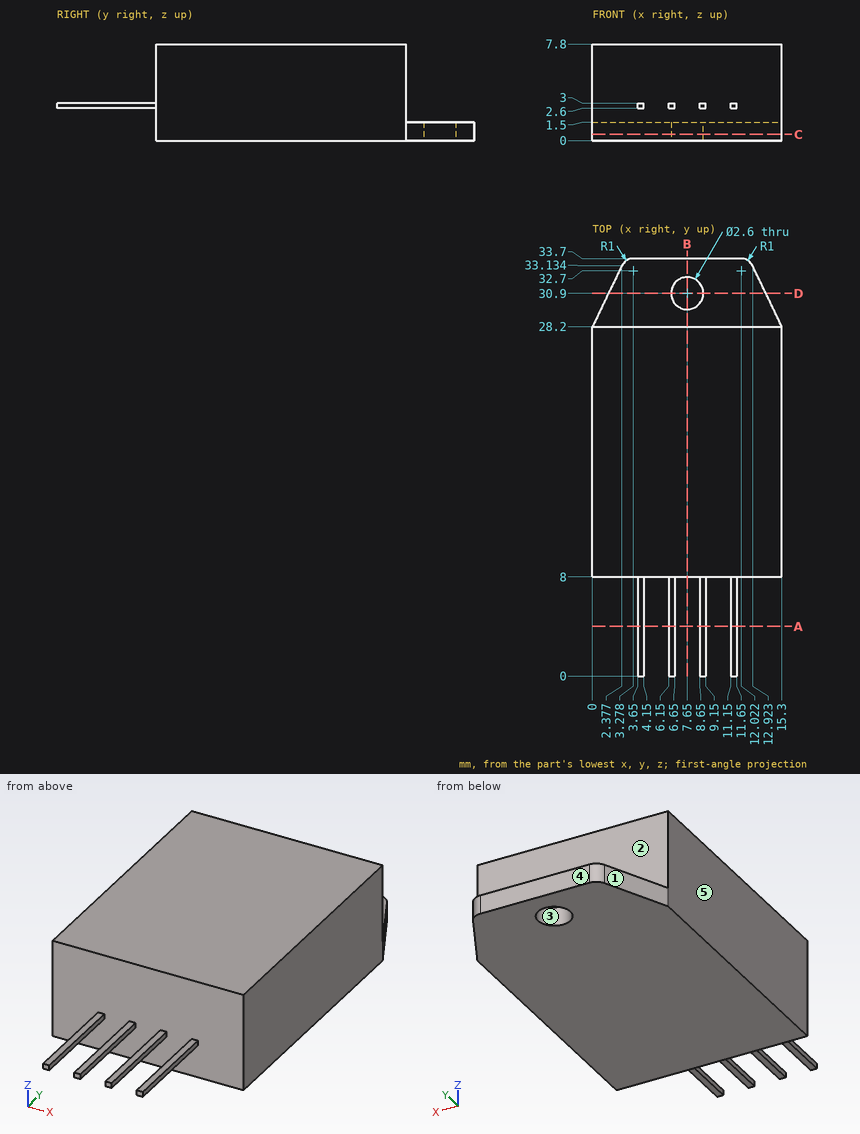
Can you work these out from the drawing? Everything is in mm from the part's minimum corner. A direction names the side the tool comes from. Round coordinates to 2 decimals unless told otherwise and drop trailing zeros. Write each loop counter-clockwise with the first axis right and the second up, starting at its lowest first coordinate (ties: lowest second). Pieces come first, ordered by that corner, then holes. Notation, with made-up numbers: (19.25, 24) - (45.25, 24) arc R18 ccw to (45.25, 44) - close; hole circle Ø4 at (12.25, 38.25). An arc over 180 degrees is marked (long way). Use a Markdown table: item, result.
Q1. Thinking about a two-plate mould opening in Y: for the marked faces 3, 4 and 5, which applies, released by +Y, released by -Y, zero draft, split by the parting line, or undercut?
Output values:
| item | result |
|---|---|
| face 3 | undercut |
| face 4 | released by +Y |
| face 5 | zero draft |
Q2. I want a section at B-B (x = 7.65). List the corners of the cut face in (y, z) for me.
Output values:
| item | result |
|---|---|
| outline | (8, 0) - (29.6, 0) - (29.6, 1.5) - (28.2, 1.5) - (28.2, 7.8) - (8, 7.8) - close; (32.2, 0) - (33.7, 0) - (33.7, 1.5) - (32.2, 1.5) - close |
Q3. Please list where these lines run through material, in increasing order: L1, parallel to Y at x = 7.65, z = 1; L2, parallel to Z at x = 8, y = 28.5; L3, parallel to Y at x = 8.75, z = 4.
Output values:
| item | result |
|---|---|
| L1 | 8 to 29.6, 32.2 to 33.7 |
| L2 | 0 to 1.5 |
| L3 | 8 to 28.2 |
Q4. For pin 1 (3 mm diameter, centred on x = 10.5, z = 4.5, fed in from -Y); pin 2 (1.5 mm diameter, centred on x = 3, z = 3.5, fed in from +Y), each with a flat end and sliding along its axis, tell me the tip position at first contact or that it passes through.
Output values:
| item | result |
|---|---|
| pin 1 | y = 8 |
| pin 2 | y = 28.2 |
Q5. I want a section at C-C (z = 0.5). List the corners of the cut face in (x, y) for me, plus the area to 3 significant figures.
Output values:
| item | result |
|---|---|
| outline | (0, 8) - (15.3, 8) - (15.3, 28.2) - (12.92, 33.13) arc R1 ccw to (12.02, 33.7) - (3.28, 33.7) arc R1 ccw to (2.38, 33.13) - (0, 28.2) - close; hole circle Ø2.6 at (7.65, 30.9) |
| area | 373 mm2 |
Q6. For the marked faces 1 and 2, which set-ups out of +Z, -Z, +X, -X, +Y, -Y let a thin tool reach every point of the face, with its end or its side?
Output values:
| item | result |
|---|---|
| face 1 | +Z, -Z, -X, +Y |
| face 2 | +Z, +X, -X, +Y |
Q7. I want a section at D-D (y = 30.9). List the corners of the cut face in (x, z) for me.
Output values:
| item | result |
|---|---|
| outline | (1.3, 0) - (6.35, 0) - (6.35, 1.5) - (1.3, 1.5) - close; (8.95, 0) - (14, 0) - (14, 1.5) - (8.95, 1.5) - close |
Q8. I want a section at A-A (y = 4). List the corners of the cut face in (x, z) for me.
Output values:
| item | result |
|---|---|
| outline | (3.65, 2.6) - (4.15, 2.6) - (4.15, 3) - (3.65, 3) - close; (6.15, 2.6) - (6.65, 2.6) - (6.65, 3) - (6.15, 3) - close; (8.65, 2.6) - (9.15, 2.6) - (9.15, 3) - (8.65, 3) - close; (11.15, 2.6) - (11.65, 2.6) - (11.65, 3) - (11.15, 3) - close |
